Check sheet for the drawn part. Datum: minimum x, y, z corner. Units: mm. A direction names the side the tool comes from. Coordinates: 2 decimals unless noted, no trailing zeros. Loops run counter-clockwise (first coordinate to the right, second up) from the corner with the lowest first, then second, coordinate; pieces in that order, holes last. Notation, with made-up numbers: (-15, 5) -> (34, 5) arc R18 ccw to (34, 40) -> close; hole circle Ø9 at (50, 33). An arc over 180 degrees is marked (long way). Use CSV: the item, a comma, the result in double quotes. Start each with the question number.
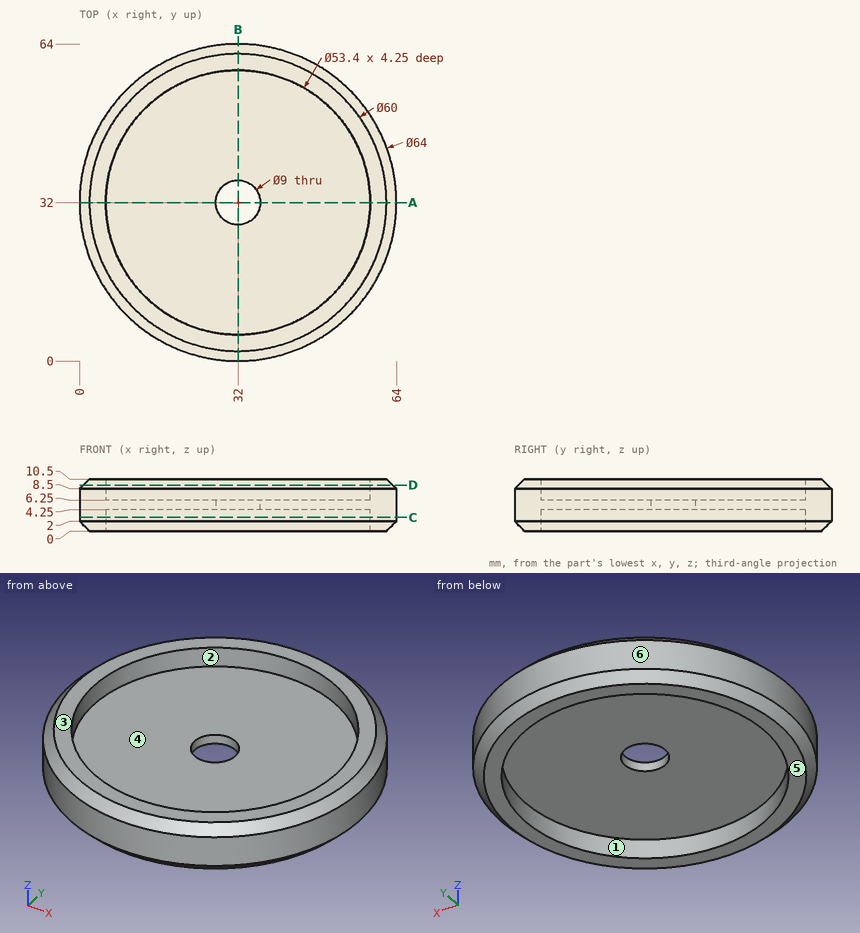
1. Scan lines: line 1 (Y direction, x = 32, z = 4.75); line 2 (Y direction, x = 32, z = 2.9); line 3 (Z direction, x = 53, y = 26.5). Record each from-to range of solid material in increasing order.
2. Set-up check for the marked faces 1, 2 and 3: record each of +Z, -Z, +X, -X, +Y, -Y from which the full face is reachable in a straight line by a thin tool's end or side.
3. Cross-section at D-D, the plane z = 9.25. Record the boundary of the cut face in (x, y), plus the area to 3 significant figures.
4. Cross-section at C-C, the plane z = 2.75. Record the boundary of the cut face in (x, y), plus the area to 3 significant figures.
5. Cross-section at A-A, the plane y = 32. Record the boundary of the cut face in (x, z), plus the area to 3 significant figures.
6. Release check for a two-part mould opening along X. For the marked faces 4, 5 and 6 record: released by +X, released by -X, zero draft, split by the parting line, or undercut.
7. Depth check by flat-ended pin: pin 1 (3 mm diameter, centred on x = 48, z = 4, fed in from +Y); pin 2 (3 mm diameter, centred on y = 12, z = 5.5, fed in from -X); pin 3 (2 mm diameter, centred on x = 13, z = 4.5, fed in from -Y). Enter the tip coordinate at first touch or a pass-through.
Solution:
1,line 1,"y = 0 to 27.5, 36.5 to 64"
1,line 2,"y = 0 to 5.3, 58.7 to 64"
1,line 3,"z = 4.25 to 6.25"
2,face 1,"-Z"
2,face 2,"+Z"
2,face 3,"+Z, +X, -X, +Y, -Y"
3,outline,"circle Ø62.5 at (32, 32); hole circle Ø53.4 at (32, 32)"
3,area,"828 mm2"
4,outline,"circle Ø64 at (32, 32); hole circle Ø53.4 at (32, 32)"
4,area,"977 mm2"
5,outline,"(0, 2) -> (2, 0) -> (5.3, 0) -> (5.3, 4.25) -> (27.5, 4.25) -> (27.5, 6.25) -> (5.3, 6.25) -> (5.3, 10.5) -> (2, 10.5) -> (0, 8.5) -> close; (36.5, 4.25) -> (58.7, 4.25) -> (58.7, 0) -> (62, 0) -> (64, 2) -> (64, 8.5) -> (62, 10.5) -> (58.7, 10.5) -> (58.7, 6.25) -> (36.5, 6.25) -> close"
5,area,"192 mm2"
6,face 4,"undercut"
6,face 5,"zero draft"
6,face 6,"split by the parting line"
7,pin 1,"stops at y = 60.53"
7,pin 2,"stops at x = 5.89"
7,pin 3,"stops at y = 5.54"
